Autodesk Inventor part; units mm, degrees
ref_plane "YZ Plane" through (0, 0, 0) normal (1, 0, 0) x (0, 1, 0)
ref_plane "XZ Plane" through (0, 0, 0) normal (0, 1, 0) x (-1, 0, 0)
ref_plane "XY Plane" through (0, 0, 0) normal (0, 0, 1) x (1, 0, 0)
sketch "Sketch1" plane through (0, 0, 0) normal (0, 0, 1) x (1, 0, 0)
  circle A0 centre (78.9796, 4.5334) radius 50
  circle A1 centre (248.9796, 4.5334) radius 30
  line L0 (78.9796, 54.5334) -> (248.9796, 34.5334)
  line L1 (248.9796, -25.4666) -> (78.9796, -45.4666)
  dimension "d25" = 170
  dimension "d26" = 100
  dimension "d27" = 60
  dimension "d28" = 0
extrude "Extrusion1" add sketch "Sketch1" along normal blind 10 contours L0 A0 L1 | L0 A1 L1 A0 | A1
sketch "Sketch2" plane through (0, 0, 10) normal (0, 0, 1) x (1, 0, 0)
  arc A0 (248.9796, -25.4666) -> (248.9796, 34.5334) centre (248.9796, 4.5334) ccw
  arc A1 (78.9796, 54.5334) -> (78.9796, -45.4666) centre (78.9796, 4.5334) ccw
hole "Hole1" at (78.9796, 4.5334, 10) at (248.9796, 4.5334, 10) direction (0, 0, -1) diameter 8 end through all
properties part number "short arm"
Can you work these out from the model? Positions are in its coordinate system, mm. Coordinates: 2 decimals unless noted, no trailing zeros. Loops run counter-clockwise (first coordinate to the right, second up) from the corner with the lowest first, then second, coordinate; pieces in that order, holes last.
1) I need wall thicknesses on probe 1 along X at (y, z) = (1, 5.5); probe 2 along X at (y, z) = (2.5, 9) (3 decimals); probe 3 along Y at (x, z) = (76, 5.75). Which ranges of each line are inside material? Lowest first, please.
2) Thinking about a two-plate mould opening in X: for faces 1 (the cylindrical face through (252.884, 5.401, 4.93)), 2 (the flat face through (162.79, 44.673, 4.93)), 3 (the cylindrical face through (75.014, 5.054, 4.93)), 4 (the flat face through (152, 5, 0)), which applies, pulls with the +X half, pulls with the -X half, needs draft (parallel to the pull), parting line crosses it, or undercut?
3) Imagine slicing it at A-A on z = 7.25. List the corners of the cut face in (x, y) for me.
4) For pin 1 (4 mm diameter, centred on y = -2, z = 2.5, fed in from +X); pin 2 (1 mm diameter, centred on x = 119, z = 2, fed in from -Y); pin 3 (5 mm diameter, centred on y = -18, z = 7.5, fed in from +X), each with a flat end and sliding along its axis, tell me the tip position at first contact or that it passes through.
5) Imagine slicing it at C-C on y = 17. List the corners of the cut face in (x, z) for me.
6) Imagine slicing it at B-B on x = 57.5. List the corners of the cut face in (y, z) for me.
Completed:
1. probe 1: x = 29.1 to 77.1, 80.85 to 247.1, 250.85 to 278.77
1. probe 2: x = 29.021 to 75.535, 82.424 to 245.535, 252.424 to 278.911
1. probe 3: y = -45.38 to 1.86, 7.2 to 54.44
2. face 1: undercut
2. face 2: pulls with the +X half
2. face 3: undercut
2. face 4: needs draft
3. outline: (78.98, -45.47) - (248.98, -25.47) arc R30 ccw to (248.98, 34.53) - (78.98, 54.53) arc R50 ccw to start; hole circle Ø8 at (78.98, 4.53); hole circle Ø8 at (248.98, 4.53)
4. pin 1: stops at x = 278.64
4. pin 2: stops at y = -40.82
4. pin 3: stops at x = 271.31
5. outline: (30.56, 0) - (276.27, 0) - (276.27, 10) - (30.56, 10) - close
6. outline: (-40.62, 0) - (49.68, 0) - (49.68, 10) - (-40.62, 10) - close
